```python
from build123d import *

# Parameters (mm, degrees)
BOX_W           = 40
BOX_H           = 8
BOX_DEPTH       = 8
SKETCH_R        = 2.5
POCKET_DEPTH    = 8
SKETCH001_R     = 1.5
POCKET001_DEPTH = 8


with BuildPart() as part:
    # Box → Box (new body)
    with BuildSketch(Plane(origin=(-20, -4, -4), x_dir=(1, 0, 0), z_dir=(0, 0, 1))):
        with Locations((20, 4)):
            Rectangle(BOX_W, BOX_H)
    extrude(amount=BOX_DEPTH)

    # Sketch → Pocket (cut)
    with BuildSketch(Plane(origin=(-20, -4, 4), x_dir=(1, 0, 0), z_dir=(0, 0, 1))):
        with Locations((26, 4)):
            Circle(SKETCH_R)
        with Locations((14, 4)):
            Circle(SKETCH_R)
    extrude(amount=-POCKET_DEPTH, mode=Mode.SUBTRACT)

    # Sketch001 → Pocket001 (cut)
    with BuildSketch(Plane(origin=(-20, -4, -4), x_dir=(1, 0, 0), z_dir=(0, -1, 0))):
        with Locations((4, 4)):
            Circle(SKETCH001_R)
        with Locations((36, 4)):
            Circle(SKETCH001_R)
    extrude(amount=-POCKET001_DEPTH, mode=Mode.SUBTRACT)


solid = part.part
```
Geometry check sheet. Reference: the model listing, model coordinates, mm. Coordinates: 2 decimals unless noted, no trailing zeros. Order: outer loops, then holes, each group sorted by start corner. A loop starts at its lowest first (then second) coordinate and runs counter-clockwise, first axis right, second up.
Q1. Depth check by flat-ended pin: pin 1 Ø4.5 at (x, y) = (6, 0) entering from -Z. Enter the tip coordinate at first touch or a pass-through.
Reply:
pin 1: passes through
Q2. Draft check along Y on faces 1 (the face through (0, -4, 0)), 2 (the face through (8.385, 0.751, 0.056)), 3 (the face through (20, 0, 0)). Enter one of: released by +Y, released by -Y, zero draft, split by the parting line, or undercut.
Reply:
face 1: released by -Y
face 2: undercut
face 3: zero draft
Q3. Sectioned sample at D-D on z = -3.25. Record the cut outline in (x, y).
Reply:
outline: (-20, -4) - (20, -4) - (20, 4) - (-20, 4) - close; hole circle Ø5 at (-6, 0); hole circle Ø5 at (6, 0)
Q4. Sectioned sample at C-C on y = -0.5. Record the cut outline in (x, z).
Reply:
outline: (-20, -4) - (-8.45, -4) - (-8.45, 4) - (-20, 4) - close; (-3.55, -4) - (3.55, -4) - (3.55, 4) - (-3.55, 4) - close; (8.45, -4) - (20, -4) - (20, 4) - (8.45, 4) - close; hole circle Ø3 at (-16, 0); hole circle Ø3 at (16, 0)
Q5. Thickness scan on probe 1 along Z at (x, y) = (16, -1); probe 2 along X at (y, z) = (-2.25, -0.25); probe 3 along X at (y, z) = (2.25, -1). Record the ranges inside material, lowest first.
Reply:
probe 1: z = -4 to -1.5, 1.5 to 4
probe 2: x = -20 to -17.48, -14.52 to -7.09, -4.91 to 4.91, 7.09 to 14.52, 17.48 to 20
probe 3: x = -20 to -17.12, -14.88 to -7.09, -4.91 to 4.91, 7.09 to 14.88, 17.12 to 20
Q6. Sectioned sample at B-B on x = -6. Record the cut outline in (y, z).
Reply:
outline: (-4, -4) - (-2.5, -4) - (-2.5, 4) - (-4, 4) - close; (2.5, -4) - (4, -4) - (4, 4) - (2.5, 4) - close
Q7. Sectioned sample at A-A on z = 0. Record the cut outline in (x, y).
Reply:
outline: (-20, -4) - (-17.5, -4) - (-17.5, 4) - (-20, 4) - close; (-14.5, -4) - (14.5, -4) - (14.5, 4) - (-14.5, 4) - close; (17.5, -4) - (20, -4) - (20, 4) - (17.5, 4) - close; hole circle Ø5 at (-6, 0); hole circle Ø5 at (6, 0)
